Could you check a few things on this model? Use its own coordinates, in mm. A direction names the side the tool comes from. Give positions to 0.01 mm unless a question says otherwise; leave off trailing zeros. Order: outer loops, then holes, each group sorted by start corner. A loop starts at its lowest first (then second) coordinate and runs counter-clockwise, first axis right, second up.
(1) Will these pins go through, and if not, where does the flat tip stop? pin 1 (1.5 mm diameter, centred on x = 4, z = 2.5, fed in from +Y); pin 2 (1 mm diameter, centred on y = 2, z = 1.5, fed in from -X).
(2) Imagine slicing it at A-A, the plane x = 6.5. Write out the boundary of the cut face in (y, z) (3 decimals), then the cut area to 3 significant figures.
(3) On a 3-axis mill with a long thin cutter (end or side, diameter ignored), from which of +Z, -Z, +X, -X, +Y, -Y can I reach the whole of each face in a straight line? I mean faces 4 (the cylindrical face through (-18.67, 6.26, 1.57)), 5 (the cylindrical face through (-22.36, 18.6, 1.57)). Say none if no direction works.
(4) Imagine slicing it at C-C, the plane y = 9.5. Write out the boundary of the cut face in (x, z) (3 decimals).
(5) If we mould it in two halves opening along X, with no side actions, what happens to faces 1 (the flat face through (-11, -15, 0)), 2 (the flat face through (-29.356, -15, 2)), 3 (the cylindrical face through (-18.76, -36.72, 1.57))? For each: released by +X, released by -X, zero draft, split by the parting line, or undercut.
(6) If I drill on probe 1 along Y at (x, z) = (0, 1.6); probe 2 along X at (y, z) = (-11.5, 1.9); probe 3 along X at (y, z) = (-6, 2.95), over which ranges is the centre line in solid material (lowest first)?
(7) Imagine slicing it at B-B, the plane z = 2.15. Write out the boundary of the cut face in (x, y).
from build123d import *

# Parameters (mm, degrees)
F0_R     = 11.938
F1_DEPTH = 3.175


# Not quite as in the source:
# - a feature names something its author has since deleted; it is built from what else it names


with BuildPart() as f1:
    # F0 (on Top) → F1 (new body)
    with BuildSketch(Plane.XY):
        with BuildLine():
            ThreePointArc((19.6894808556, 0.0781131055), (13.8950303962, 13.9502648114), (0, 19.6896358021))
            Line((0, 19.6896358021), (-20.0037127642, 19.6896358021))
            ThreePointArc((-20.0037127642, 19.6896358021), (-22.390015477, 18.5774210568), (-24.1276545988, 16.5995250638))
            ThreePointArc((-24.1276545988, 16.5995250638), (-28.0183229898, 8.6377085048), (-29.3558392303, -0.1223641979))
            Line((-29.3558392303, -0.1223641979), (-29.3558392303, -30.3483641979))
            ThreePointArc((-29.3558392303, -30.3483641979), (-28.5482645978, -37.1866304526), (-26.1699732087, -43.6486573967))
            ThreePointArc((-26.1699732087, -43.6486573967), (-25.2069369553, -45.3941485327), (-24.1276545988, -47.0702534596))
            ThreePointArc((-24.1276545988, -47.0702534596), (-22.390015477, -49.0481494526), (-20.0037127642, -50.1603641979))
            Line((-20.0037127642, -50.1603641979), (0, -50.1603641979))
            ThreePointArc((0, -50.1603641979), (13.9381398986, -44.4282647716), (19.8109856608, -30.5488415012))
            Line((19.8109856608, -30.5488415012), (19.6894808556, 0.0781131055))
        make_face()
        with BuildLine():
            Line((-19.6805191444, 0.5991028516), (-19.8109856608, -30.5488415012))
            ThreePointArc((-19.8109856608, -30.5488415012), (-18.7320573688, -36.8001368793), (-15.7326179982, -42.3899618877))
            ThreePointArc((-15.7326179982, -42.3899618877), (-15.4201129826, -44.616632299), (-16.6477696645, -46.5003996883))
            ThreePointArc((-16.6477696645, -46.5003996883), (-19.2439967199, -47.0478700205), (-21.3627294259, -45.4506566945))
            ThreePointArc((-21.3627294259, -45.4506566945), (-24.9332630835, -38.2716109559), (-26.1619083245, -30.3483641979))
            Line((-26.1619083245, -30.3483641979), (-26.1434258244, 0.1322556929))
            ThreePointArc((-26.1434258244, 0.1322556929), (-24.8969528592, 7.9773393892), (-21.3520418939, 15.0859707133))
            ThreePointArc((-21.3520418939, 15.0859707133), (-19.3084814881, 16.3545849229), (-16.9550367483, 15.8577761045))
            ThreePointArc((-16.9550367483, 15.8577761045), (-15.5712636207, 13.7334477776), (-16.1488403601, 11.2648441198))
            ThreePointArc((-16.1488403601, 11.2648441198), (-18.6915825929, 6.1892243613), (-19.6805191444, 0.5991028516))
        make_face(mode=Mode.SUBTRACT)
        with Locations((0, -30.3483641979)):
            Circle(F0_R, mode=Mode.SUBTRACT)
        with BuildLine():
            ThreePointArc((-15.3116747346, 7.469335274), (0, 17.0363832022), (15.3116747346, 7.469335274))
            ThreePointArc((15.3116747346, 7.469335274), (15.6883641196, -6.6418057683), (5.2940419625, -16.1929451402))
            ThreePointArc((5.2940419625, -16.1929451402), (0, -15.2353641979), (-5.2940419625, -16.1929451402))
            ThreePointArc((-5.2940419625, -16.1929451402), (-15.6883641196, -6.6418057683), (-15.3116747346, 7.469335274))
        make_face(mode=Mode.SUBTRACT)
    extrude(amount=F1_DEPTH)


solid = f1.part
Answer block:
1. pin 1: stops at y = 19.42
1. pin 2: stops at x = -29.31
2. outline: (-49.064, 0) - (-40.362, 0) - (-40.362, 3.175) - (-49.064, 3.175) - close; (-20.335, 0) - (-15.748, 0) - (-15.748, 3.175) - (-20.335, 3.175) - close; (15.748, 0) - (18.586, 0) - (18.586, 3.175) - (15.748, 3.175) - close
2. area: 51.2 mm2
3. face 4: +Z, -Z
3. face 5: +Z, -Z, -X, +Y
4. outline: (-27.734, 0) - (-24.357, 0) - (-24.357, 3.175) - (-27.734, 3.175) - close; (-17.246, 0) - (-14.142, 0) - (-14.142, 3.175) - (-17.246, 3.175) - close; (14.142, 0) - (17.246, 0) - (17.246, 3.175) - (14.142, 3.175) - close
5. face 1: zero draft
5. face 2: released by -X
5. face 3: undercut
6. probe 1: y = -50.16 to -42.29, -18.41 to -15.24, 17.04 to 19.69
6. probe 2: x = -29.36 to -26.15, -19.73 to -12.57, 12.57 to 19.74
6. probe 3: x = -29.36 to -26.15, -19.71 to -15.94, 15.94 to 19.71
7. outline: (-29.36, -30.35) arc R29.36 ccw to (-24.13, -47.07) arc R6.41 ccw to (-20, -50.16) - (0, -50.16) arc R19.81 ccw to (19.81, -30.55) - (19.69, 0.08) arc R19.69 ccw to (0, 19.69) - (-20, 19.69) arc R6.41 ccw to (-24.13, 16.6) arc R29.36 ccw to (-29.36, -0.12) - close; hole (-26.16, -30.35) arc R26.16 ccw to (-21.36, -45.45) arc R3.2 ccw to (-15.73, -42.39) arc R19.81 cw to (-19.81, -30.55) - (-19.68, 0.6) arc R19.69 cw to (-16.15, 11.26) arc R3.23 ccw to (-21.35, 15.09) arc R26.14 ccw to (-26.14, 0.13) - close; hole circle Ø23.88 at (0, -30.35); hole (-5.29, -16.19) arc R15.11 cw to (5.29, -16.19) arc R17.04 ccw (long way) to start
